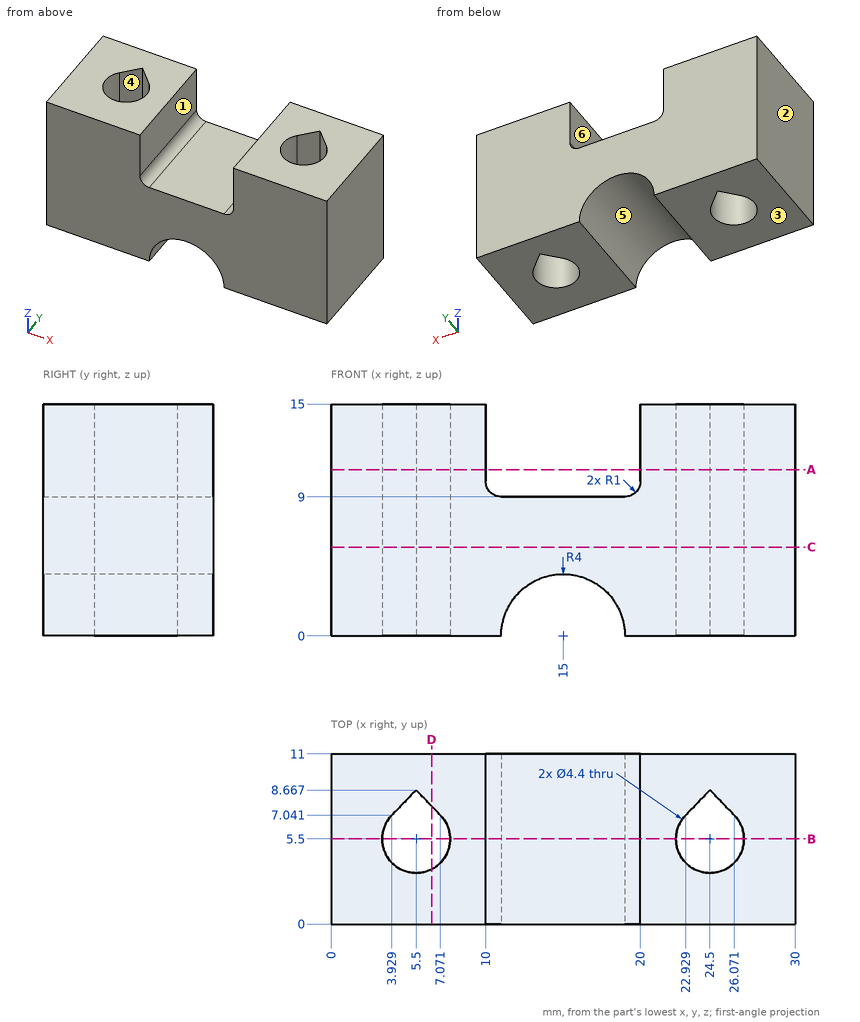
Part print with two shaded views. Sizes in mm from the minimum x, y, z corner. A direction names the side the tool comes from. Round coordinates to 2 decimals unless told otherwise and drop trailing zeros. Order: outer loops, then holes, each group sorted by start corner. A loop starts at its lowest first (then second) coordinate and runs counter-clockwise, first axis right, second up. Notation, with made-up numbers: (37.5, -7.5) -> (64.5, -7.5) arc R29 ccw to (64.5, 24.5) -> close; hole circle Ø6 at (26, 42). An arc over 180 degrees is marked (long way). Use one line per item in the form item = value.
Item 1: Pull direction X, two halves, no side cores. Call the marked faces 1, 2 and 3: released by +X, released by -X, zero draft, split by the parting line, or undercut.
Returned:
face_1 = undercut
face_2 = released by -X
face_3 = zero draft
Item 2: Flat gauge pins, fed straight in: pin 1 Ø4 at (x, y) = (13, 4.5) entering from +Z; pin 2 Ø5 at (x, y) = (24.5, 7) entering from +Z; pin 3 Ø1 at (x, y) = (16, 6.5) entering from -Z. Where does each tip first touch, or does it go through?
Returned:
pin_1 = 9
pin_2 = 15
pin_3 = 3.71
Item 3: Tool access for the marked faces 4, 5 and 6: list every direction of +Z, -Z, +X, -X, +Y, -Y with a clear straight run to the whole face (end or side of a thin tool).
Returned:
face_4 = +Z, -Z
face_5 = -Z, +Y, -Y
face_6 = +Z, +Y, -Y
Item 4: Drill centre lines: line 1 (X direction, y = 5.5, z = 5.25); line 2 (X direction, y = 4.75, z = 14.5); line 3 (X direction, y = 8.5, z = 3) (1 decimal). Where is each one in solid material? Low to high.
Returned:
line_1 = 0 to 3.3, 7.7 to 22.3, 26.7 to 30
line_2 = 0 to 3.43, 7.57 to 10, 20 to 22.43, 26.57 to 30
line_3 = 0 to 5.3, 5.7 to 12.4, 17.6 to 24.3, 24.7 to 30
Item 5: Cut at B-B, the plane y = 5.5. Write the cut outline in (x, z).
Returned:
outline = (0, 0) -> (3.3, 0) -> (3.3, 15) -> (0, 15) -> close; (7.7, 0) -> (11, 0) arc R4 cw to (19, 0) -> (22.3, 0) -> (22.3, 15) -> (20, 15) -> (20, 10) arc R1 cw to (19, 9) -> (11, 9) arc R1 cw to (10, 10) -> (10, 15) -> (7.7, 15) -> close; (26.7, 0) -> (30, 0) -> (30, 15) -> (26.7, 15) -> close
Item 6: Cut at C-C, the plane z = 5.75. Write the cut outline in (x, y).
Returned:
outline = (0, 0) -> (30, 0) -> (30, 11) -> (0, 11) -> close; hole (3.93, 7.04) arc R2.2 ccw (long way) to (7.07, 7.04) -> (5.5, 8.67) -> close; hole (22.93, 7.04) arc R2.2 ccw (long way) to (26.07, 7.04) -> (24.5, 8.67) -> close
Item 7: Cut at A-A, the plane z = 10.75. Write the cut outline in (x, y).
Returned:
outline = (0, 0) -> (10, 0) -> (10, 11) -> (0, 11) -> close; (20, 0) -> (30, 0) -> (30, 11) -> (20, 11) -> close; hole (3.93, 7.04) arc R2.2 ccw (long way) to (7.07, 7.04) -> (5.5, 8.67) -> close; hole (22.93, 7.04) arc R2.2 ccw (long way) to (26.07, 7.04) -> (24.5, 8.67) -> close
Item 8: Cut at D-D, the plane x = 6.5. Write the cut outline in (y, z), and give its area (3 significant figures).
Returned:
outline = (0, 0) -> (3.54, 0) -> (3.54, 15) -> (0, 15) -> close; (7.63, 0) -> (11, 0) -> (11, 15) -> (7.63, 15) -> close
area = 104 mm^2
